from build123d import *

# Parameters (mm, degrees)
SKETCH_1_W        = 280
SKETCH_1_H        = 200
EXTRUDE_1_DEPTH   = 120
EXTRUDE_START     = -90
EXTRUDE_1_2_DEPTH = 30


with BuildPart() as part:
    # 草图1 → Extrude 1 (new body)
    with BuildSketch(Plane(origin=(0, 0, 0), x_dir=(1, 0, 0), z_dir=(0, 1, 0))):
        with Locations((140, 100)):
            Rectangle(SKETCH_1_W, SKETCH_1_H)
    extrude(amount=EXTRUDE_1_DEPTH)

    # 草图2 → Extrude 1 2 (add)
    with BuildSketch(Plane.XY.offset(EXTRUDE_START)):
        with BuildLine():
            ThreePointArc((56.840474866, 120), (141.048835122, 137.874678511), (225.257195379, 120))
            Line((225.257195379, 120), (221.194887056, 110.862295086))
            ThreePointArc((221.194887056, 110.862295086), (141.048835122, 127.874678511), (60.902783189, 110.862295086))
            Line((60.902783189, 110.862295086), (56.840474866, 120))
        make_face()
    extrude(amount=-EXTRUDE_1_2_DEPTH)


solid = part.part
Could you check a few things on this model? Use its own coordinates, in mm. A direction names the side the tool comes from. Give positions to 0.01 mm unless a question says otherwise; leave off trailing zeros. Order: outer loops, then holes, each group sorted by start corner. A loop starts at its lowest first (then second) coordinate and runs counter-clockwise, first axis right, second up.
1. I need wall thicknesses on L1, parallel to Y at x = 254.5, z = -147.5. Which ranges of the line are inside material? Lowest first, please.
Answers below:
L1: y = 0 to 120
2. Thinking about a two-plate mould opening in X: for faces 3 (the cylindrical face through (141.832, 127.873, -104.79)), 4 (the flat face through (0, 59, -99)), 5 (the flat face through (142, 129, -120)), which applies, +X half, -X half, draft (parallel to the pull), parting line (faces both ways), or undercut?
Answers below:
face 3: undercut
face 4: -X half
face 5: draft
3. Suppose I cut it at C-C (z = -144). Write out the boundary of the cut face in (x, y).
Answers below:
outline: (0, 0) - (280, 0) - (280, 120) - (0, 120) - close
4. Which directions (+Z, -Z, +X, -X, +Y, -Y) give clear straight access to the entire face, cutting with the end or side of a thin tool? Please do faces 1 (the flat face through (280, 59, -99)), 2 (the flat face through (142, 129, -90)).
Answers below:
face 1: +Z, -Z, +X, +Y, -Y
face 2: +Z, +X, -X, +Y
5. Suppose I cut it at B-B (x = 199.5). Write out the boundary of the cut face in (y, z).
Answers below:
outline: (0, -200) - (120, -200) - (120, -120) - (129.46, -120) - (129.46, -90) - (120, -90) - (120, 0) - (0, 0) - close
6. For pin 1 (8 mm diameter, centred on x = 238.5, z = -67, fed in from -Y); pin 2 (19.5 mm diameter, centred on x = 120.5, y = 130.5, fed in from +Z); pin 3 (9 mm diameter, centred on x = 156, y = 132, fed in from -Z), each with a flat end and sliding along its axis, tell me the tip position at first contact or that it passes through.
Answers below:
pin 1: stops at y = 0
pin 2: stops at z = -90
pin 3: stops at z = -120
7. Suppose I cut it at A-A (x = 136). Write out the boundary of the cut face in (y, z), plus the area to 3 significant figures.
Answers below:
outline: (0, -200) - (120, -200) - (120, 0) - (0, 0) - close; (127.81, -120) - (137.81, -120) - (137.81, -90) - (127.81, -90) - close
area: 24,300 mm2
8. Suppose I cut it at D-D (x = 79.5). Write out the boundary of the cut face in (y, z).
Answers below:
outline: (0, -200) - (120, -200) - (120, -120) - (128.53, -120) - (128.53, -90) - (120, -90) - (120, 0) - (0, 0) - close
